```python
from build123d import *

# Parameters (mm, degrees)
CROQUIS1_W              = 12
CROQUIS1_H              = 22.9
SALIENTE_EXTRUIR1_DEPTH = 5
VACIADO2_T              = -1
CROQUIS2_R              = 2.28
SALIENTE_EXTRUIR2_DEPTH = 4
CROQUIS4_R              = 1
CORTAR_EXTRUIR1_DEPTH   = 0.8
CROQUIS5_R              = 0.4
CORTAR_EXTRUIR2_DEPTH   = 0.8


with BuildPart() as part:
    # Croquis1 → Saliente-Extruir1 (new body)
    with BuildSketch(Plane(origin=(0, 0, 0), x_dir=(0, 0, -1), z_dir=(1, 0, 0))):
        with Locations((-17.987585454, -24.1598532)):
            Rectangle(CROQUIS1_W, CROQUIS1_H)
    extrude(amount=SALIENTE_EXTRUIR1_DEPTH)

    # Vaciado2
    vaciado2_openings = [part.faces().sort_by_distance(p)[0] for p in [
        (5, -24.1598532, 17.987585454),
    ]]
    offset(amount=VACIADO2_T, openings=vaciado2_openings, kind=Kind.INTERSECTION)

    # Croquis2 → Saliente-Extruir2 (add)
    with BuildSketch(Plane.ZY):
        with Locations((17.987585454, -17.75436054)):
            Circle(CROQUIS2_R)
    extrude(amount=SALIENTE_EXTRUIR2_DEPTH)

    # Croquis4 → Cortar-Extruir1 (cut)
    with BuildSketch(Plane.ZY):
        with Locations((13.487585454, -14.2098532)):
            Circle(CROQUIS4_R)
        with Locations((22.487585454, -14.2098532)):
            Circle(CROQUIS4_R)
        with Locations((13.487585454, -34.1098532)):
            Circle(CROQUIS4_R)
        with Locations((22.487585454, -34.1098532)):
            Circle(CROQUIS4_R)
    extrude(amount=-CORTAR_EXTRUIR1_DEPTH, mode=Mode.SUBTRACT)

    # Croquis5 → Cortar-Extruir2 (cut)
    with BuildSketch(Plane.ZY.offset(-0.8)):
        with Locations((13.487585454, -14.2098532)):
            Circle(CROQUIS5_R)
        with Locations((22.487585454, -14.2098532)):
            Circle(CROQUIS5_R)
        with Locations((13.487585454, -34.1098532)):
            Circle(CROQUIS5_R)
        with Locations((22.487585454, -34.1098532)):
            Circle(CROQUIS5_R)
    extrude(amount=-CORTAR_EXTRUIR2_DEPTH, mode=Mode.SUBTRACT)


solid = part.part
```
Model file for the job. Use its own axes, mm. A direction names the side the tool comes from. Coordinates: 2 decimals unless noted, no trailing zeros. Loops run counter-clockwise (first coordinate to the right, second up) from the corner with the lowest first, then second, coordinate; pieces in that order, holes last. Notation, with made-up numbers: (62, 11) - (101, 11) arc R25 cw to (101, 39) - close; hole circle Ø4 at (29, -14.5). An arc over 180 degrees is marked (long way). Answer as a JSON object with one key per item and string values. Group by question number.
(1) Cut at D-D (y = -17.25). Give the cut face in (x, z), then the cut area to 3 significant figures.
(2) Probe line 1 along Z through (x, y) = (0.25, -14.25); line 2 along Z through (x, y) = (4.25, -15.5); line 3 along Y through (x, z) = (0.75, 22). List the from-to ranges inside material, lowest first.
(3) Cut at C-C (z = 21). Give the cut face in (x, y), then the cut area to 3 significant figures.
(4) Flat gauge pins, fed straight in: pin 1 (5 mm diameter, centred on y = -23.5, z = 16, fed in from -X); pin 2 (1.6 mm diameter, centred on y = -34, z = 22.5, fed in from -X). Where does each tip first touch, or does it go through?
(5) Tool access for faces 5 (the face through (2, -24, 11.988)), 6 (the face through (0.394, -14.818, 21.694)), 7 (the face through (3, -13.71, 18)): list every direction of +Z, -Z, +X, -X, +Y, -Y with a clear straight run to the whole face (end or side of a thin tool).
(6) Cut at B-B (y = -30.25). Give the cut face in (x, z).
(7) Cut at A-A (x = 2.75). Give the cut face in (y, z), then the cut area to 3 significant figures.
(8) Two-plate mould, pull along Z, no slides. Class faces 1 (the face through (0.8, -14, 23)), 2 (the face through (-1.97, -19.98, 17.49)), 3 (the face through (2, -35.61, 18)), 4 (the face through (3, -24, 22.988)): released by +Z, released by -Z, zero draft, split by the parting line, or undercut.
Geometry says:
{
 "1": {"outline": "(-4, 15.76) - (0, 15.76) - (0, 11.99) - (5, 11.99) - (5, 12.99) - (1, 12.99) - (1, 22.99) - (5, 22.99) - (5, 23.99) - (0, 23.99) - (0, 20.21) - (-4, 20.21) - close", "area": "37.8 mm^2"},
 "2": {"line 1": "z = 11.99 to 12.49, 14.49 to 21.49, 23.49 to 23.99", "line 2": "z = 11.99 to 12.99, 22.99 to 23.99", "line 3": "y = -35.61 to -34.98, -33.24 to -15.08, -13.34 to -12.71"},
 "3": {"outline": "(0, -35.61) - (5, -35.61) - (5, -34.61) - (1, -34.61) - (1, -13.71) - (5, -13.71) - (5, -12.71) - (0, -12.71) - close", "area": "30.9 mm^2"},
 "4": {"pin 1": "stops at x = 0", "pin 2": "stops at x = 0.8"},
 "5": {"face 5": "-Z, +X, -X, +Y, -Y", "face 6": "-X", "face 7": "+X"},
 "6": {"outline": "(0, 11.99) - (5, 11.99) - (5, 12.99) - (1, 12.99) - (1, 22.99) - (5, 22.99) - (5, 23.99) - (0, 23.99) - close"},
 "7": {"outline": "(-35.61, 11.99) - (-12.71, 11.99) - (-12.71, 23.99) - (-35.61, 23.99) - close; hole (-34.61, 12.99) - (-13.71, 12.99) - (-13.71, 22.99) - (-34.61, 22.99) - close", "area": "65.8 mm^2"},
 "8": {"face 1": "undercut", "face 2": "split by the parting line", "face 3": "zero draft", "face 4": "undercut"}
}
